Drawing for the job (mm, zero at the part's lowest x, y, z). A direction names the side the tool comes from. Round coordinates to 2 decimals unless told otherwise and drop trailing zeros. Write each loop counter-clockwise with the first axis right and the second up, starting at its lowest first coordinate (ties: lowest second). Pieces come first, ordered by that corner, then holes.
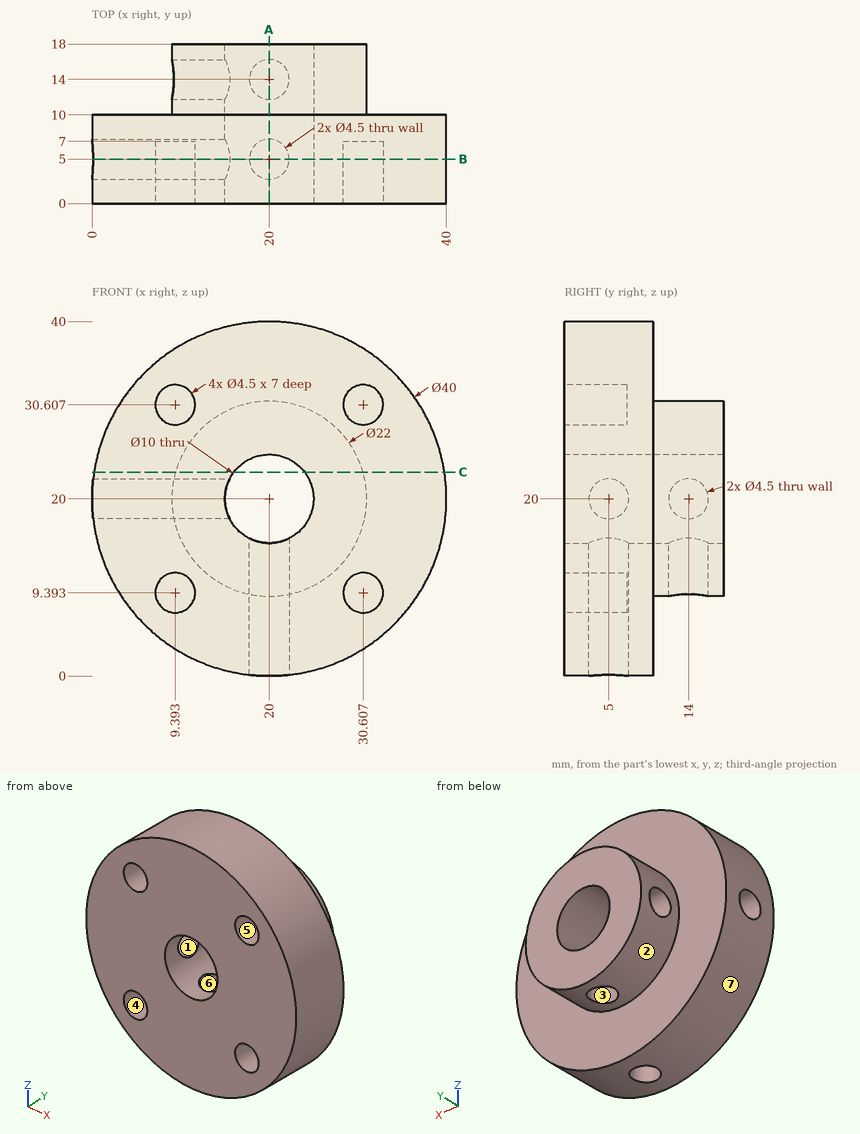
1) Wall check: probe 1 along Y at (x, z) = (8.5, 13); probe 2 along Z at (x, y) = (8, 3.75) (1 decimal); probe 3 along X at (y, z) = (4.5, 14) (1 decimal). Give the ranges that are in metal, low to high.
2) Pull direction Z, two halves, no side cores. Call the marked faces 5, 6 and 7: released by +Z, released by -Z, zero draft, split by the parting line, or undercut.
3) Which spindle directions (+Z, -Z, +X, -X, +Y, -Y) get a long thin tool onto all of the face, cutting with end or side? Do the marked faces 1, 2, 3 and 4. Say none if no direction does.
4) Flat gauge pins, fed straight in: pin 1 Ø1.3 at (x, z) = (9.5, 9) entering from -Y; pin 2 Ø2.5 at (x, z) = (9.39, 9.39) entering from +Y; pin 3 Ø8 at (y, z) = (15, 31) entering from -X (1 decimal). Where does each tip first touch, or does it go through?
5) Cut at C-C on z = 23. List the corners of the cut face in (x, y), and give its area (3 significant figures).
6) Cut at A-A on x = 20. List the corners of the cut face in (y, z).
7) Cut at B-B on y = 5. Give the number of separate pieces and of enclosed holes in the cut face, and give its area (3 significant figures).
Result sheet:
1. probe 1: y = 0 to 10
1. probe 2: z = 4 to 7.6, 11.2 to 18.1, 21.9 to 28.8, 32.4 to 36
1. probe 3: x = 0.9 to 17.8, 22.2 to 39.1
2. face 5: undercut
2. face 6: zero draft
2. face 7: split by the parting line
3. face 1: -X
3. face 2: +Y
3. face 3: -Z
3. face 4: -Y
4. pin 1: stops at y = 7
4. pin 2: stops at y = 10
4. pin 3: stops at x = 11.5
5. outline: (0.23, 0) - (16, 0) - (16, 18) - (9.42, 18) - (9.42, 10) - (0.23, 10) - close; (24, 0) - (39.77, 0) - (39.77, 10) - (30.58, 10) - (30.58, 18) - (24, 18) - close
5. area: 421 mm2
6. outline: (0, 0) - (2.75, 0) - (2.75, 15) - (0, 15) - close; (0, 25) - (18, 25) - (18, 31) - (10, 31) - (10, 40) - (0, 40) - close; (7.25, 0) - (10, 0) - (10, 9) - (11.75, 9) - (11.75, 15) - (7.25, 15) - close; (16.25, 9) - (18, 9) - (18, 15) - (16.25, 15) - close
7. separate pieces: 2
7. enclosed holes: 4
7. area: 978 mm2
